Check sheet for the modelled part. Datum: model origin and axes. Units: mm. Round coordinates to 2 decimals unless told otherwise and drop trailing zeros. Order: outer loops, then holes, each group sorted by start corner. A loop starts at its lowest first (then second) coordinate and runs counter-clockwise, first axis right, second up.
Autodesk Inventor part; units mm, degrees
ref_plane "YZ Plane" through (0, 0, 0) normal (1, 0, 0) x (0, 1, 0)
ref_plane "XZ Plane" through (0, 0, 0) normal (0, 1, 0) x (-1, 0, 0)
ref_plane "XY Plane" through (0, 0, 0) normal (0, 0, 1) x (1, 0, 0)
sketch "Náčrt1" plane through (0, 0, 0) normal (0, 1, 0) x (-1, 0, 0)
  line L0 (0, 0) -> (178, 0)
  line L1 (178, 0) -> (178, 178)
  line L2 (178, 178) -> (0, 178)
  line L3 (0, 178) -> (0, 0)
  circle A0 centre (9, 9) radius 2
  circle A1 centre (169, 169) radius 2
  circle A2 centre (9, 169) radius 2
  circle A3 centre (169, 9) radius 2
  line L4 (163, 163) -> (157, 169)
  line L5 (163, 15) -> (169, 21)
  line L6 (21, 9) -> (157, 9)
  line L7 (15, 15) -> (21, 9)
  line L8 (15, 15) -> (9, 21)
  line L9 (169, 21) -> (157, 9)
  line L10 (21, 169) -> (9, 157)
  line L11 (9, 157) -> (9, 21)
  line L12 (157, 169) -> (21, 169)
  line L13 (169, 21) -> (169, 157)
  line L14 (163, 163) -> (169, 157)
  dimension "d0" = 178
  dimension "d1" = 178
  dimension "d37" = 9
  dimension "d38" = 9
extrude "Vysunutí1" add sketch "Náčrt1" against normal blind 10
sketch "Náčrt2" plane through (0, -10, 0) normal (0, -1, 0) x (1, 0, 0)
  line L0 (-3, 3) -> (-175, 3)
  line L1 (-175, 3) -> (-175, 175)
  line L2 (-175, 175) -> (-3, 175)
  line L3 (-3, 175) -> (-3, 3)
  line L4 (-178, 0) -> (0, 0)
  line L5 (0, 0) -> (0, 178)
  line L6 (-178, 0) -> (0, 0)
  line L7 (0, 0) -> (0, 178)
  line L8 (0, 178) -> (-178, 178)
  line L9 (-178, 178) -> (-178, 0)
  dimension "d68" = 172
  dimension "d69" = 172
extrude "Vysunutí2" add sketch "Náčrt2" along normal blind 3
sketch "Náčrt3" plane through (0, 0, 0) normal (0, 1, 0) x (1, 0, 0)
  line L0 (-3, -3) -> (-175, -3)
  line L1 (-175, -3) -> (-175, -175)
  line L2 (-175, -175) -> (-3, -175)
  line L3 (-3, -175) -> (-3, -3)
  line L4 (-169, -21) -> (-157, -9)
  line L5 (-157, -9) -> (-169, -21)
  line L6 (-169, -21) -> (-169, -157)
  line L7 (-175, -175) -> (-175, -3)
  line L8 (-169, -157) -> (-157, -169)
  line L9 (-21, -169) -> (-157, -169)
  line L10 (-157, -169) -> (-21, -169)
  line L11 (-9, -157) -> (-9, -21)
  line L12 (-21, -169) -> (-9, -157)
  line L13 (-21, -9) -> (-9, -21)
  line L14 (-9, -157) -> (-9, -21)
  line L15 (-9, -21) -> (-21, -9)
  line L16 (-157, -9) -> (-21, -9)
  line L17 (-21, -9) -> (-157, -9)
  circle A0 centre (-9, -9) radius 2
  circle A1 centre (-9, -169) radius 2
  circle A2 centre (-9, -169) radius 2
  circle A3 centre (-169, -9) radius 2
  circle A4 centre (-169, -169) radius 2
extrude "Vysunutí4" add sketch "Náčrt3" along normal blind 3
properties part number "Cougar_Base"
Item 1: Release check for a two-part mould opening along Z. For faces 1 (the flat face through (-89, -10, 172)), 2 (the flat face through (-178, -6, 88)), 3 (the flat face through (-88, -6, 0)), 4 (the flat face through (-90, -6, 178)) record: released by +Z, released by -Z, zero draft, split by the parting line, or undercut.
Answer:
face 1: undercut
face 2: zero draft
face 3: released by -Z
face 4: released by +Z
Item 2: Sectioned sample at A-A (z = 14.5). Record the cut outline in (x, y), and give its area (3 significant figures).
Answer:
outline: (-178, -13) - (-175, -13) - (-175, -10) - (-162.5, -10) - (-162.5, 3) - (-175, 3) - (-175, 0) - (-178, 0) - close; (-15.5, -10) - (-3, -10) - (-3, -13) - (0, -13) - (0, 0) - (-3, 0) - (-3, 3) - (-15.5, 3) - close
area: 403 mm2
Item 3: Sectioned sample at C-C (x = -96). Record the cut outline in (y, z), and give its area (3 significant figures).
Answer:
outline: (-13, 0) - (0, 0) - (0, 3) - (3, 3) - (3, 9) - (-10, 9) - (-10, 3) - (-13, 3) - close; (-13, 175) - (-10, 175) - (-10, 169) - (3, 169) - (3, 175) - (0, 175) - (0, 178) - (-13, 178) - close
area: 234 mm2
Item 4: Go/stop test with flat-tipped pins: P1, Ø0.9, axis at x = -64.5, y = 1.5, coming from the +Z side; P2, Ø2, axis at y = 1.5, z = 25, coming from the -X side; P3, Ø0.9, axis at y = 1, z = 109, coming from the +X side. Record where each tip stops, or that it passes through.
Answer:
P1: stops at z = 175
P2: stops at x = -175
P3: stops at x = -3
Item 5: Scan lines: line 1 along X through (y, z) = (-7, 75); line 2 along Z through (x, y) = (-114, -0.75); line 3 along X through (y, z) = (-10.25, 53). Record each from-to range of solid material in increasing order.
Answer:
line 1: x = -178 to -169, -9 to 0
line 2: z = 0 to 9, 169 to 178
line 3: x = -178 to -175, -3 to 0
Item 6: Sectioned sample at B-B (y = -4.25). Record the cut outline in (x, z).
Answer:
outline: (-178, 0) - (0, 0) - (0, 178) - (-178, 178) - close; hole circle Ø4 at (-169, 9); hole circle Ø4 at (-169, 169); hole (-169, 21) - (-157, 9) - (-21, 9) - (-9, 21) - (-9, 157) - (-21, 169) - (-157, 169) - (-169, 157) - close; hole circle Ø4 at (-9, 9); hole circle Ø4 at (-9, 169)
